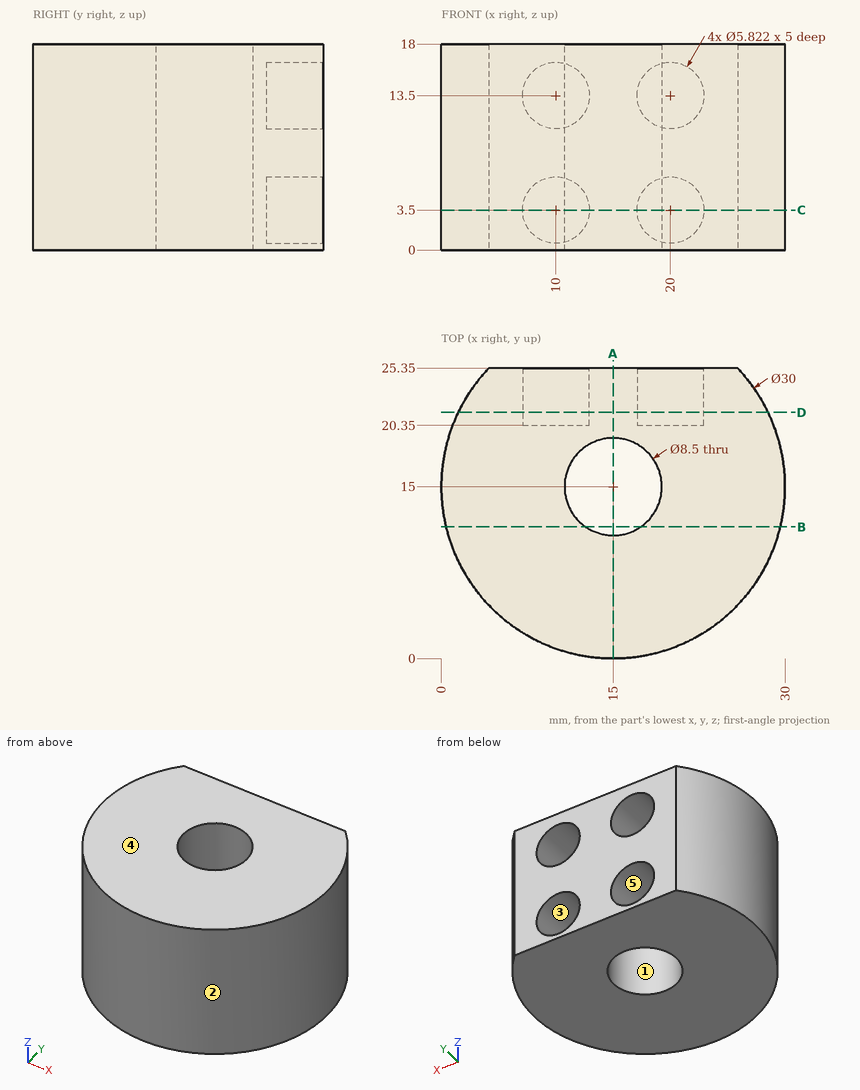
Study the drawing (mm; zero at the part's minimum x, y, z) and answer. A direction names the side the tool comes from. Round coordinates to 2 decimals unless told otherwise and drop trailing zeros. Write each loop counter-clockwise with the first axis right and the second up, starting at its lowest first coordinate (ties: lowest second). Pieces come first, ordered by that corner, then holes. Notation, with made-up numbers: (-14, -20) - (-8, -20) arc R25 cw to (-8, 11) - close; hole circle Ø2 at (-21, -2). An arc over 180 degrees is marked (long way). Return JSON: item names as keys, results as strings. Group by question number.
Q1. Each of these flat-tipped pins is pushed along its axis until it touches: pin 1 Ø1.7 at (x, z) = (21, 3) entering from +Y; pin 2 Ø5 at (x, y) = (14.5, 16) entering from -Z; pin 3 Ø9.5 at (x, z) = (20, 13.5) entering from -Y; pin 4 Ø1.5 at (x, z) = (7.5, 9.5) entering from -Y (1 decimal). Where does it stop, or does it pass through?
Q2. The part is cut by section B-B on y = 11.5. Write down the section's boundary in (x, z), then the cut area to 3 significant figures.
Q3. The part is cut by section C-C on z = 3.5. Write down the section's boundary in (x, y).
Q4. Find the intervals of material crossed by L1, parallel to Z at x = 10, y = 24.15; L2, parallel to X at y = 23, z = 12.25; L3, parallel to Z at x = 17.5, y = 22.5, in increasing order.
Q5. For the marked faces 4 and 5, determine the directions among +Z, -Z, +X, -X, +Y, -Y from which every point of the face is accessible in a straight line to the end or side of a thin tool.
Q6. The mould has two halves that part along Y. Classify the marked faces 1, 2 and 3: released by +Y, released by -Y, zero draft, split by the parting line, or undercut.
Q7. The part is cut by section D-D on y = 21.5. Write down the section's boundary in (x, z).
Q8. The part is cut by section A-A on x = 15. Write down the section's boundary in (y, z), then the cut area to 3 significant figures.
Solved:
{
 "1": {"pin 1": "y = 20.35", "pin 2": "through", "pin 3": "y = 0", "pin 4": "y = 1.6"},
 "2": {"outline": "(0.41, 0) - (12.59, 0) - (12.59, 18) - (0.41, 18) - close; (17.41, 0) - (29.59, 0) - (29.59, 18) - (17.41, 18) - close", "area": "438 mm²"},
 "3": {"outline": "(4.14, 25.35) arc R15 ccw (long way) to (25.86, 25.35) - (22.91, 25.35) - (22.91, 20.35) - (17.09, 20.35) - (17.09, 25.35) - (12.91, 25.35) - (12.91, 20.35) - (7.09, 20.35) - (7.09, 25.35) - close; hole circle Ø8.5 at (15, 15)"},
 "4": {"L1": "0 to 0.59, 6.41 to 10.59, 16.41 to 18", "L2": "2.31 to 7.37, 12.63 to 17.37, 22.63 to 27.69", "L3": "0 to 2.01, 4.99 to 12.01, 14.99 to 18"},
 "5": {"face 4": "+Z, +X, -X, +Y, -Y", "face 5": "+Y"},
 "6": {"face 1": "undercut", "face 2": "split by the parting line", "face 3": "zero draft"},
 "7": {"outline": "(1.48, 0) - (28.52, 0) - (28.52, 18) - (1.48, 18) - close; hole circle Ø5.82 at (10, 3.5); hole circle Ø5.82 at (10, 13.5); hole circle Ø5.82 at (20, 3.5); hole circle Ø5.82 at (20, 13.5)"},
 "8": {"outline": "(0, 0) - (10.75, 0) - (10.75, 18) - (0, 18) - close; (19.25, 0) - (25.35, 0) - (25.35, 18) - (19.25, 18) - close", "area": "303 mm²"}
}
